For this review, take the finished solid that the model builds, in its own axes (mm). Give positions to 0.01 mm unless a question says otherwise; leave off trailing zeros. Loops run counter-clockwise (first coordinate to the right, second up) from the corner with the lowest first, then second, coordinate; pieces in that order, holes last. Notation, with made-up numbers: M 18,27.5 L 66,27.5 A34 cw 66,62.5 Z; hole C -38,19.5 d5. An arc over 180 degrees is marked long. Use CSV: the item, a comma, the result in double quotes. Start each with the question number.
1. Take a section at B-B, the plane x = 29. Write out the cut boundary in (y, z).
2. Take a section at C-C, the plane y = -21. Write out the cut boundary in (x, z), and give its area (3 significant figures).
3. Take a section at A-A, the plane z = 2.5. Write out the cut boundary in (x, y), and give its area (3 significant figures).
4. To check wall thickness, follow line 1 (X direction, y = -3.5, z = 5.5); line 2 (Y direction, x = -26, z = 5); line 3 (Y direction, x = 25, z = 3.5). State the ranges of each line that lie inside material, in increasing order. Write a range as [from, to].
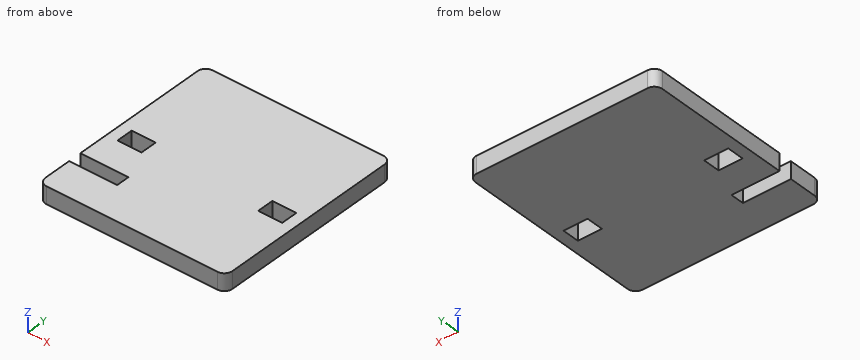
from build123d import *

# Parameters (mm, degrees)
SKETCH1_W           = 70
SKETCH1_H           = 73.5
BOSS_EXTRUDE1_DEPTH = 6.35
SKETCH2_W           = 9
SKETCH2_H           = 6.35
SKETCH2_W_2         = 17.9920326
SKETCH2_H_2         = 5
CUT_EXTRUDE1_DEPTH  = 6.35
FILLET1_R           = 3


with BuildPart() as part:
    # Sketch1 → Boss-Extrude1 (new body)
    with BuildSketch(Plane.XY):
        Rectangle(SKETCH1_W, SKETCH1_H)
    extrude(amount=BOSS_EXTRUDE1_DEPTH)

    # Sketch2 → Cut-Extrude1 (cut)
    with BuildSketch(Plane.XY.offset(6.35)):
        with Locations((-26.35, -3.575)):
            Rectangle(SKETCH2_W, SKETCH2_H)
        with Locations((-26.0039837, -20.75)):
            Rectangle(SKETCH2_W_2, SKETCH2_H_2)
        with Locations((26.35, -3.575)):
            Rectangle(SKETCH2_W, SKETCH2_H)
    extrude(amount=-CUT_EXTRUDE1_DEPTH, mode=Mode.SUBTRACT)

    # Fillet1
    fillet1_edges = [part.edges().sort_by_distance(p)[0] for p in [
        (35, -36.75, 3.175),
        (-35, -36.75, 3.175),
        (-35, 36.75, 3.175),
        (35, 36.75, 3.175),
    ]]
    fillet(fillet1_edges, radius=FILLET1_R)


solid = part.part
Result set:
1,outline,"M -36.75,0 L -6.75,0 L -6.75,6.35 L -36.75,6.35 Z; M -0.4,0 L 36.75,0 L 36.75,6.35 L -0.4,6.35 Z"
2,outline,"M -17.01,0 L 35,0 L 35,6.35 L -17.01,6.35 Z"
2,area,"330 mm2"
3,outline,"M -35,-33.75 A3 ccw -32,-36.75 L 32,-36.75 A3 ccw 35,-33.75 L 35,33.75 A3 ccw 32,36.75 L -32,36.75 A3 ccw -35,33.75 L -35,-18.25 L -17.01,-18.25 L -17.01,-23.25 L -35,-23.25 Z; hole M -30.85,-6.75 L -21.85,-6.75 L -21.85,-0.4 L -30.85,-0.4 Z; hole M 21.85,-6.75 L 30.85,-6.75 L 30.85,-0.4 L 21.85,-0.4 Z"
3,area,"4,930 mm2"
4,line 1,"[-35, -30.85], [-21.85, 21.85], [30.85, 35]"
4,line 2,"[-36.75, -23.25], [-18.25, -6.75], [-0.4, 36.75]"
4,line 3,"[-36.75, -6.75], [-0.4, 36.75]"
